```python
from build123d import *

# Parameters (mm, degrees)
BOSS_EXTRUDE1_DEPTH             = 6
CUT_EXTRUDE1_DEPTH              = 1
CUT_EXTRUDE2_DEPTH              = 4.5
M5X0_8_TAPPED_HOLE1_D           = 4.2
M5X0_8_TAPPED_HOLE1_CSINK_D     = 5.05
M5X0_8_TAPPED_HOLE1_CSINK_ANGLE = 90


with BuildPart() as part:
    # Sketch1 → Boss-Extrude1 (new body)
    with BuildSketch(Plane.XY):
        Polygon((-3, 4.5), (3, 4.5), (3, 3.5), (5, 3.5), (5, 2.5), (2.5, 0), (-2.5, 0), (-5, 2.5), (-5, 3.5), (-3, 3.5), align=None)
    extrude(amount=BOSS_EXTRUDE1_DEPTH)

    # Sketch2 → Cut-Extrude1 (cut)
    with BuildSketch(Plane(origin=(0, 4.5, 0), x_dir=(1, 0, 0), z_dir=(0, 1, 0))):
        with BuildLine():
            Line((0, -6), (3, -6))
            Line((3, -6), (3, -3))
            ThreePointArc((3, -3), (2.121320344, -5.121320344), (0, -6))
        make_face()
        with BuildLine():
            Line((0, 0), (-3, 0))
            Line((-3, 0), (-3, -3))
            ThreePointArc((-3, -3), (-2.121320344, -0.878679656), (0, 0))
        make_face()
    extrude(amount=-CUT_EXTRUDE1_DEPTH, mode=Mode.SUBTRACT)

    # Sketch3 → Cut-Extrude2 (cut, through all)
    with BuildSketch(Plane(origin=(0, 3.5, 0), x_dir=(1, 0, 0), z_dir=(0, 1, 0))):
        with BuildLine():
            Line((5, -3), (5, -6))
            Line((5, -6), (3.5, -6))
            ThreePointArc((3.5, -6), (4.604101966, -4.677050983), (5, -3))
        make_face()
        with BuildLine():
            Line((-5, 0), (-3.5, 0))
            ThreePointArc((-3.5, 0), (-4.604101966, -1.322949017), (-5, -3))
            Line((-5, -3), (-5, 0))
        make_face()
    extrude(amount=-CUT_EXTRUDE2_DEPTH, mode=Mode.SUBTRACT)

    # M5x0.8 Tapped Hole1 (through all)
    with Locations(Plane(origin=(0, 4.5, 0), x_dir=(1, 0, 0), z_dir=(0, 1, 0))):
        with Locations((0, -3)):
            CounterSinkHole(M5X0_8_TAPPED_HOLE1_D / 2, M5X0_8_TAPPED_HOLE1_CSINK_D / 2, counter_sink_angle=M5X0_8_TAPPED_HOLE1_CSINK_ANGLE)


solid = part.part
```
Could you check a few things on this model? Use its own coordinates, in mm. A direction names the side the tool comes from. Round coordinates to 2 decimals unless told otherwise and drop trailing zeros. Write each loop counter-clockwise with the first axis right and the second up, starting at its lowest first coordinate (ties: lowest second). Pieces come first, ordered by that corner, then holes.
(1) Suppose I cut it at D-D on x = 4.5. Write out the boundary of the cut face in (y, z), and give its area (3 significant figures).
Findings below:
outline: (2, 0) - (3.5, 0) - (3.5, 4.87) - (2, 4.87) - close
area: 7.31 mm2
(2) If I drill on probe 1 along Z at (x, y) = (0, 2.25); probe 2 along Z at (x, y) = (-1, 3.3); probe 3 along X at (y, z) = (1.2, 3.2), over which ranges is the centre line in solid material (lowest first)?
Findings below:
probe 1: z = 0 to 0.9, 5.1 to 6
probe 2: z = 0 to 1.15, 4.85 to 6
probe 3: x = -3.7 to -2.09, 2.09 to 3.7
(3) Suppose I cut it at A-A on y = 3.85. Write out the boundary of the cut face in (x, z), and give its area (3 significant figures).
Findings below:
outline: (-3, 3) arc R3 ccw to (0, 0) - (3, 0) - (3, 3) arc R3 ccw to (0, 6) - (-3, 6) - close; hole circle Ø4.2 at (0, 3)
area: 18.3 mm2
(4) Thinking about a two-plate mould opening in Z: for faces 1 (the face through (2.14, 4.01, 5.1)), 2 (the face through (1, 2, 0)), 3 (the face through (-0.969, 2.009, 4.863)), 4 (the face through (3.8, 1.3, 3)), which applies, +Z half, -Z half, draft (parallel to the pull), parting line (faces both ways), or undercut?
Findings below:
face 1: +Z half
face 2: -Z half
face 3: undercut
face 4: draft
(5) Suppose I cut it at C-C on y = 3.4. Write out the boundary of the cut face in (x, z).
Findings below:
outline: (-5, 3) arc R3.75 ccw to (-3.5, 0) - (5, 0) - (5, 3) arc R3.75 ccw to (3.5, 6) - (-5, 6) - close; hole circle Ø4.2 at (0, 3)
(6) For pin 1 (0.8 mm diameter, centred on y = 4, z = 5, fed in from -X); pin 2 (3 mm diameter, centred on x = -3.5, z = 5, fed in from +Y), each with a flat end and sliding along its axis, tell me the tip position at first contact or that it passes through.
Findings below:
pin 1: stops at x = -3
pin 2: stops at y = 4.5
(7) Which directions (+Z, -Z, +X, -X, +Y, -Y) give clear straight access to the entire face, cutting with the end or side of a thin tool? Please do faces 5 (the face through (-2.14, 4.01, 0.9)), 6 (the face through (-3, 4, 4)), 7 (the face through (3, 4, 1)), 8 (the face through (-5, 3, 4)).
Findings below:
face 5: -Z, -X, +Y
face 6: +Z, -Z, -X, +Y
face 7: +Z, -Z, +X, +Y
face 8: +Z, -Z, -X, +Y, -Y
